Autodesk Inventor part; units mm, degrees
ref_plane "YZ Plane" through (0, 0, 0) normal (1, 0, 0) x (0, 1, 0)
ref_plane "XZ Plane" through (0, 0, 0) normal (0, 1, 0) x (-1, 0, 0)
ref_plane "XY Plane" through (0, 0, 0) normal (0, 0, 1) x (1, 0, 0)
sketch "Sketch1" plane through (0, 0, 0) normal (0, 0, 1) x (1, 0, 0)
  circle A0 centre (0, 0) radius 14.2875
  line L0 (0, 0) -> (-24.2467, 24.2467) construction
  line L1 (0, 0) -> (34.29, 0) construction
  circle A1 centre (-24.2467, 24.2467) radius 11.1125
  line L2 (-24.2467, 24.2467) -> (8.7733, 24.2467) construction
  line L3 (-24.2467, 24.2467) -> (0, 24.2467) construction
  line L4 (0, 24.2467) -> (0, 46.6502) construction
  line L5 (0, 46.6502) -> (-24.2467, 24.2467) construction
  circle A2 centre (0, 46.6502) radius 11.1125
  line L6 (0, 46.6502) -> (-25.4, 46.6502) construction
  line L7 (-25.4, 46.6502) -> (25.4, 46.6502) construction
  circle A3 centre (-25.4, 46.6502) radius 2.5797
  circle A4 centre (25.4, 46.6502) radius 2.5797
  line L8 (0, 46.6502) -> (0, 65.7002) construction
  line L9 (0, 65.7002) -> (44.45, 65.7002)
  line L10 (44.45, 65.7002) -> (44.45, -39.0748)
  line L11 (0, 65.7002) -> (-44.45, 65.7002)
  line L12 (-44.45, 65.7002) -> (-44.45, -39.0748)
  line L13 (-44.45, -39.0748) -> (44.45, -39.0748)
  dimension "d0" = 28.575
  dimension "d1" = 34.29
  dimension "d2" = 135
  dimension "d3" = 22.225
  dimension "d7" = 22.4035
  dimension "d8" = 22.225
  dimension "d9" = 25.4
  dimension "d10" = 50.8
  dimension "d11" = 5.1594
  dimension "d12" = 19.05
  dimension "d13" = 104.775
  dimension "d14" = 44.45
  dimension "d17" = 44.45
  dimension "d23" = 5.1594
extrude "Extrusion1" add sketch "Sketch1" along normal blind 6.35
sketch "Sketch2" plane through (0, 0, 6.35) normal (0, 0, 1) x (1, 0, 0)
  line L0 (-44.45, 65.7002) -> (-39.37, 65.7002) construction
  line L1 (-44.45, 65.7002) -> (44.45, 65.7002) construction
  line L2 (-39.37, 65.7002) -> (-39.37, 60.6202) construction
  circle A0 centre (-39.37, 60.6202) radius 2.5797
  line L3 (0, 65.7002) -> (0, -39.0748) construction
  line L4 (-44.45, -39.0748) -> (44.45, -39.0748) construction
  line L5 (44.45, -39.0748) -> (44.45, 65.7002) construction
  line L6 (44.45, 13.3127) -> (-44.45, 13.3127) construction
  circle A1 centre (39.37, 60.6202) radius 2.5797
  circle A2 centre (-39.37, -33.9948) radius 2.5797
  circle A3 centre (39.37, -33.9948) radius 2.5797
  point P0 (0, 0)
  dimension "d18" = 5.08
  dimension "d19" = 5.08
  dimension "d20" = 5.1594
extrude "Extrusion2" cut sketch "Sketch2" against normal blind 25.4
sketch "Sketch3" plane through (0, 0, 6.35) normal (0, 0, 1) x (1, 0, 0)
  line L0 (44.45, 65.7002) -> (44.45, -39.0748) construction
  line L1 (44.45, 0) -> (44.45, 6.35) construction
  line L2 (44.45, 6.35) -> (57.15, 6.35)
  line L3 (57.15, 6.35) -> (57.15, -6.35)
  line L4 (57.15, -6.35) -> (44.45, -6.35)
  line L5 (44.45, -6.35) -> (44.45, 6.35)
  circle A0 centre (50.8, 0) radius 2.5797
  line L6 (0, 18.1836) -> (0, -18.812) construction
  line L7 (-44.45, 65.7002) -> (-44.45, -39.0748) construction
  line L8 (-44.45, 0) -> (-44.45, 6.35) construction
  line L9 (-44.45, 6.35) -> (-57.15, 6.35)
  line L10 (-57.15, 6.35) -> (-57.15, -6.35)
  line L11 (-57.15, -6.35) -> (-44.45, -6.35)
  line L12 (-44.45, -6.35) -> (-44.45, 6.35)
  circle A1 centre (-50.8, 0) radius 2.5797
  point P0 (0, 0)
  dimension "d24" = 6.35
  dimension "d25" = 12.7
  dimension "d26" = 12.7
  dimension "d27" = 5.1594
extrude "Extrusion3" add sketch "Sketch3" against normal blind 6.35
fillet "Fillet1" radius 3.175 4 edges at (44.45, 6.35, 3.175) (44.45, -6.35, 3.175) (-44.45, -6.35, 3.175) (-44.45, 6.35, 3.175)
properties part number "Gearbox Plate"
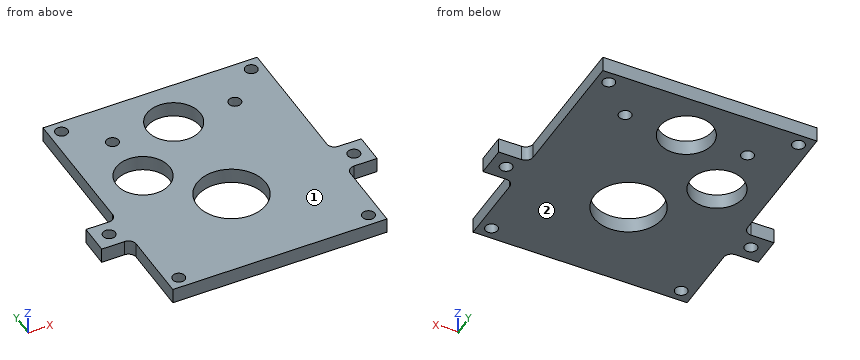
Geometry check sheet. Reference: the model listing, model coordinates, mm. Face numbers are marked on the shaded views. Coordinates: 2 decimals unless noted, no trailing zeros. Loops run counter-clockwise (first coordinate to the right, second up) from the corner with the lowest first, then second, coordinate; pieces in that order, holes last.
Item 1: Sectioned sample at B-B, the plane x = 0. Record the boundary of the cut face in (y, z).
Item 2: Sectioned sample at C-C, the plane y = 21. Record the boundary of the cut face in (x, z), then the cut area to 3 significant figures.
Item 3: Sectioned sample at A-A, the plane x = -50.8. Record the boundary of the cut face in (y, z).
Item 4: Release check for a two-part mould opening along Z. For the marked faces 1 and 2 record: released by +Z, released by -Z, zero draft, split by the parting line, or undercut.
Item 5: Thickness scan on line 1 (Y direction, x = 39.37, z = 5.25); line 2 (X direction, y = 61, z = 3); line 3 (Y direction, x = 6.5, z = 5.75). Record the ranges inside material, lowest first.
Item 6: Sectioned sample at D-D, the plane z = 1.25. Count the separate pieces of the cut face and the enclosed holes in it, then the cut area to 3 significant figures.
Item 7: Go/stop test with flat-tipped pins: pin 1 Ø3 at (x, z) = (50.5, 4.5) entering from -Y; pin 2 Ø1 at (y, z) = (16.5, 1) entering from +X; pin 3 Ø20 at (x, y) = (0, 46.65) entering from +Z; pin 4 Ø1 at (y, z) = (-13, 5) entering from -X. Record where each tip stops, or that it passes through.
Check result:
1. outline: (-39.07, 0) - (-14.29, 0) - (-14.29, 6.35) - (-39.07, 6.35) - close; (14.29, 0) - (35.54, 0) - (35.54, 6.35) - (14.29, 6.35) - close; (57.76, 0) - (65.7, 0) - (65.7, 6.35) - (57.76, 6.35) - close
2. outline: (-44.45, 0) - (-34.87, 0) - (-34.87, 6.35) - (-44.45, 6.35) - close; (-13.62, 0) - (44.45, 0) - (44.45, 6.35) - (-13.62, 6.35) - close
2. area: 430 mm2
3. outline: (-6.35, 0) - (-2.58, 0) - (-2.58, 6.35) - (-6.35, 6.35) - close; (2.58, 0) - (6.35, 0) - (6.35, 6.35) - (2.58, 6.35) - close
4. face 1: released by +Z
4. face 2: released by -Z
5. line 1: y = -39.07 to -36.57, -31.42 to 58.04, 63.2 to 65.7
5. line 2: x = -44.45 to -41.92, -36.82 to 36.82, 41.92 to 44.45
5. line 3: y = -39.07 to -12.72, 12.72 to 37.64, 55.66 to 65.7
6. separate pieces: 1
6. enclosed holes: 11
6. area: 8,060 mm2
7. pin 1: stops at y = -6.35
7. pin 2: stops at x = 44.45
7. pin 3: passes through
7. pin 4: stops at x = -44.45
